Answer from the drawing. Dimensions are ordinates in mm from the lowest x, y and z of the part. A direction names the side the tool comes from. Give positions to 0.01 mm unless a question says otherwise; leave off trailing zeros. Loops run counter-clockwise (first coordinate to the right, second up) from the corner with the lowest first, then second, coordinate; pieces in that order, holes last. Notation, with made-up numbers: (0, 40.25) - (14, 40.25) arc R19 ccw to (14, 73.25) - close; hole circle Ø5 at (78.5, -24). An arc over 180 degrees is marked (long way). Answer as CSV lines item,"result". Start each with the question number.
1) For a pull along Z with two mould halves and no side action, classify the marked faces 1, 2, 3 and 4 as pulls with the +Z half, pulls with the -Z half, needs draft (parallel to the pull), parting line crosses it, or undercut.
2) Find the intervals of material crossed by line 1 along Z through (x, y) = (25.5, 34.5) (1 decimal); line 2 along Z through (x, y) = (11, 57); line 3 along X through (y, z) = (41, 29.5) (1 decimal), in increasing order.
3) A cutting plane is placed at C-C (x = 29.5). Determine the outline of the cut face in (y, z).
4) Flat-ended cylindrical pins translate along their axes: pin 1 (3 mm diameter, centred on x = 23, y = 20, fed in from +Z); pin 2 (11.5 mm diameter, centred on x = 19.59, y = 60, fed in from +Z); pin 3 (8 mm diameter, centred on x = 19.59, y = 60, fed in from -Z). Find the tip coordinate at first contact, or state that the pin passes through.
5) A cutting plane is placed at A-A (z = 29). Determine the outline of the cut face in (x, y).
6) A cutting plane is placed at D-D (y = 33). Determine the outline of the cut face in (x, z) (1 decimal).
7) A cutting plane is placed at B-B (y = 58.5). Determine the outline of the cut face in (x, z) (1 decimal).
8) For the marked faces 5 and 6, determine the directions among +Z, -Z, +X, -X, +Y, -Y from which every point of the face is accessible in a straight line to the end or side of a thin tool.
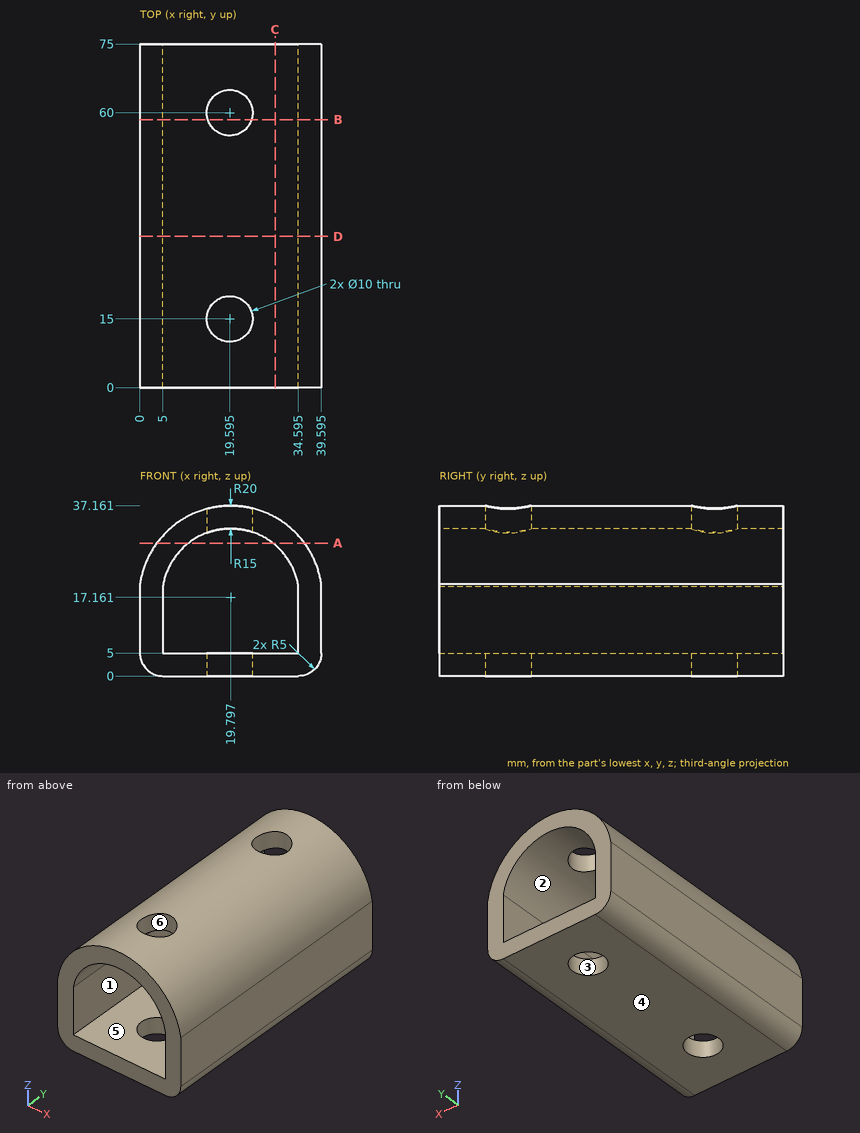
Ans:
1,face 1,"undercut"
1,face 2,"undercut"
1,face 3,"needs draft"
1,face 4,"pulls with the -Z half"
2,line 1,"0 to 5, 31 to 36.3"
2,line 2,"0 to 5, 29.31 to 35.12"
2,line 3,"4.1 to 11.3, 28.3 to 35.5"
3,outline,"(0, 0) - (75, 0) - (75, 5) - (0, 5) - close; (0, 28.6) - (75, 28.6) - (75, 34.65) - (0, 34.65) - close"
4,pin 1,"z = 37.09"
4,pin 2,"z = 37.16"
4,pin 3,"through"
5,outline,"(3.68, 0) - (10.59, 0) - (10.59, 75) - (3.68, 75) - close; (29.01, 0) - (35.92, 0) - (35.92, 75) - (29.01, 75) - close"
6,outline,"(0, 5) arc R5 ccw to (5, 0) - (34.6, 0) arc R5 ccw to (39.6, 5) - (39.6, 20) arc R20 ccw to (0, 20) - close; hole (5, 5) - (34.6, 5) - (34.6, 19.6) arc R15 ccw to (5, 19.6) - close"
7,outline,"(0, 5) arc R5 ccw to (5, 0) - (14.8, 0) - (14.8, 5) - (5, 5) - (5, 19.6) arc R15 cw to (14.8, 31.3) - (14.8, 36.5) arc R20 ccw to (0, 20) - close; (24.4, 0) - (34.6, 0) arc R5 ccw to (39.6, 5) - (39.6, 20) arc R20 ccw to (24.4, 36.6) - (24.4, 31.4) arc R15 cw to (34.6, 19.6) - (34.6, 5) - (24.4, 5) - close"
8,face 5,"+Y, -Y"
8,face 6,"+Z, -Z"
